Geometry check sheet. Reference: the model listing, model coordinates, mm. Face numbers are marked on the shaded views. Give positions to 0.01 mm unless a question says otherwise; leave off trailing zeros. Order: outer loops, then holes, each group sorted by start corner. A loop starts at its lowest first (then second) coordinate and runs counter-clockwise, first axis right, second up. Notation, with made-up numbers: (85, -12) - (96, -12) arc R18 ccw to (96, -3) - close; hole circle Ø7 at (18.5, 16.25). An arc over 180 degrees is marked (long way). Put each result on its own line as item: value. Start each with the question number.
```python
from build123d import *

# Parameters (mm, degrees)
DIAPROFILES_R         = 3
DIAPROFILES_R_2       = 2.5
DIAPROFILE_DEPTH      = 1
BEARINGPATHPROFILES_R = 0.5


with BuildPart() as part:
    # DiaProfileS → DiaProfile (new body, symmetric)
    with BuildSketch(Plane(origin=(0, 0, 0), x_dir=(1, 0, 0), z_dir=(0, 1, 0))):
        Circle(DIAPROFILES_R)
        Circle(DIAPROFILES_R_2, mode=Mode.SUBTRACT)
    extrude(amount=DIAPROFILE_DEPTH, both=True)

    # BearingPathProfileS → BearingPathProfile (revolve, cut)
    with BuildSketch(Plane.XY):
        with Locations((2.125, 0)):
            Circle(BEARINGPATHPROFILES_R)
    revolve(axis=Axis((0, 1, 0), (0, -1, 0)), mode=Mode.SUBTRACT)


solid = part.part
```
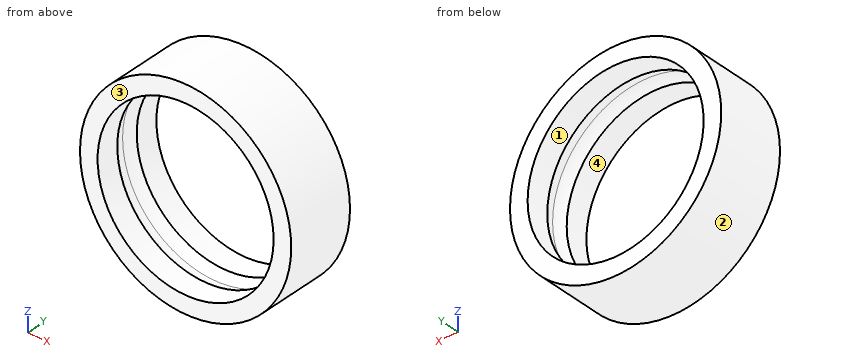
Item 1: Cross-section at A-A (x = 0). Enter the section's corners in (y, z) (3 decimals).
Item 2: Thickness scan on line 1 along X through (y, z) = (0.8, 0); line 2 along X through (y, z) = (0, 1.65). Record the ranges inside material, lowest first.
Item 3: Cross-section at D-D (y = 0.2). Enter the section's corners in (x, z).
Item 4: Cross-section at C-C (y = 0.6). Enter the section's corners in (x, z).
Item 5: Release check for a two-part mould opening along Z. For the marked faces 1, 2, 3 and 4 record: +Z half, -Z half, draft (parallel to the pull), parting line (faces both ways), or undercut.
Item 6: Cross-section at B-B (z = 0). Enter the section's corners in (x, y) (3 decimals), and give its area (3 significant figures).
Recorded:
1. outline: (-1, -3) - (1, -3) - (1, -2.5) - (0.331, -2.5) arc R0.5 cw to (-0.331, -2.5) - (-1, -2.5) - close; (-1, 2.5) - (-0.331, 2.5) arc R0.5 cw to (0.331, 2.5) - (1, 2.5) - (1, 3) - (-1, 3) - close
2. line 1: x = -3 to -2.5, 2.5 to 3
2. line 2: x = -2.51 to -2.04, 2.04 to 2.51
3. outline: circle Ø6 at (0, 0); hole circle Ø5.17 at (0, 0)
4. outline: circle Ø6 at (0, 0); hole circle Ø5 at (0, 0)
5. face 1: undercut
5. face 2: parting line
5. face 3: draft
5. face 4: undercut
6. outline: (-3, -1) - (-2.5, -1) - (-2.5, -0.331) arc R0.5 cw to (-2.5, 0.331) - (-2.5, 1) - (-3, 1) - close; (2.5, -1) - (3, -1) - (3, 1) - (2.5, 1) - (2.5, 0.331) arc R0.5 cw to (2.5, -0.331) - close
6. area: 1.89 mm^2
